For this review, take the finished solid that the model builds, in its own axes (mm). Face numbers are marked on the shaded views. A direction names the side the tool comes from. Round coordinates to 2 decimals unless told otherwise and drop trailing zeros. Order: outer loops, then holes, each group sorted by start corner. A loop starts at its lowest first (then second) coordinate and runs counter-clockwise, first axis right, second up. Notation, with made-up numbers: (14.5, 26.5) - (72.5, 26.5) arc R33 ccw to (72.5, 64.5) - close; hole circle Ø1 at (-26.75, 63). An arc over 180 degrees is marked (long way). One line per item, written item: value.
Autodesk Inventor part; units mm, degrees
ref_plane "YZ Plane" through (0, 0, 0) normal (1, 0, 0) x (0, 1, 0)
ref_plane "XZ Plane" through (0, 0, 0) normal (0, 1, 0) x (-1, 0, 0)
ref_plane "XY Plane" through (0, 0, 0) normal (0, 0, 1) x (1, 0, 0)
sketch "Sketch1" plane through (0, 0, 0) normal (0, 1, 0) x (-1, 0, 0)
  circle A0 centre (0, 0) radius 61.087
  circle A1 centre (0, 0) radius 88.9
  dimension "d0" = 122.174
  dimension "d1" = 177.8
extrude "Extrusion1" add sketch "Sketch1" along normal blind 5.08
sketch "Sketch2" plane through (0, 5.08, 0) normal (0, 1, 0) x (1, 0, 0)
  circle A0 centre (0, 0) radius 61.087
  circle A1 centre (0, 0) radius 66.167
  dimension "d4" = 132.334
  dimension "d5" = 122.174
extrude "Extrusion2" add sketch "Sketch2" along normal blind 38.354
sketch "Sketch3" plane through (0, 5.08, 0) normal (0, 1, 0) x (1, 0, 0)
  circle A0 centre (0, 0) radius 66.167
  circle A1 centre (0, 0) radius 88.9
  line L0 (66.167, 0) -> (88.9, 0) construction
  line L1 (66.167, 0) -> (77.5335, 0)
  circle A2 centre (77.5335, 0) radius 3.175
  point P0 (80.7085, 0)
  dimension "d10" = 6.35
  dimension "d8" = 22.733
  dimension "d9" = 11.3665
  dimension "d11" = 8.1915
hole "Hole1" at (77.5335, 5.08, 0) direction (0, -1, 0) diameter 6.35 end through all
pattern_circular "Circular Pattern1" count 6 over 360 about axis through (0, -10, 0) along (0, 1, 0) of "Hole1"
sketch "Sketch4" plane through (0, 5.08, 0) normal (0, 1, 0) x (1, 0, 0)
  circle A0 centre (0, 0) radius 66.167
  line L0 (43.7225, 49.663) -> (63.9658, 61.7381)
  circle A1 centre (0, 0) radius 88.9
  line L1 (64.5029, 14.7462) -> (84.7557, 26.827)
  arc A2 (64.5029, 14.7462) -> (41.6667, 51.4) centre (0, 0) ccw
  arc A3 (81.2449, 36.0899) -> (63.9658, 61.7381) centre (0, 0) ccw
  circle A4 centre (77.5335, 0) radius 3.175
  circle A5 centre (38.7668, 67.146) radius 3.175
extrude "Extrusion3" add sketch "Sketch4" along normal blind 38.354 contours A0 L0 A1 L1 picked at (52.8659, 51.2219)
sketch "Sketch5" plane through (72.0744, 43.434, -52.0431) normal (0.8107358, 0, -0.5854122) x (0, 1, 0)
  circle A0 centre (-18.8086, 0) radius 3.175
  point P0 (-43.434, 0)
  dimension "d24" = 6.35
properties part number "flangev3"
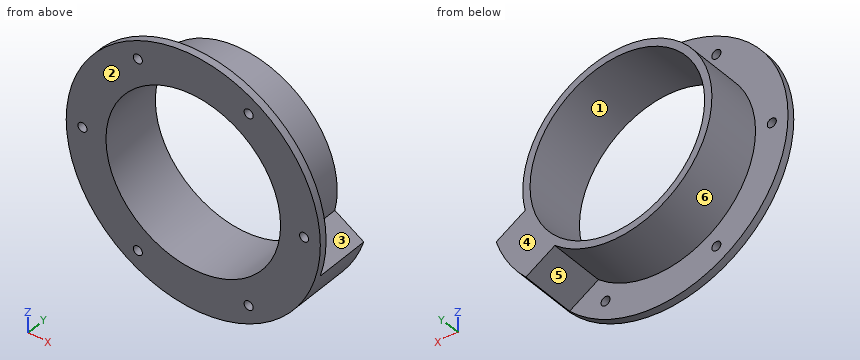
Item 1: Take a section at C-C (y = 24). Write out the cut boundary in (x, z).
Returned:
outline: (43.72, -49.66) - (63.97, -61.74) arc R88.9 ccw to (84.76, -26.83) - (64.5, -14.75) arc R66.17 ccw (long way) to start; hole circle Ø122.17 at (0, 0)
Item 2: The part is to be moulded in two halves that separate along X. For the marked faces 1, 2 and 3, say which applies: +X half, -X half, draft (parallel to the pull), parting line (faces both ways), or undercut.
Returned:
face 1: undercut
face 2: draft
face 3: +X half
Item 3: Wall thickness on line 1 (X direction, y = 3.5, z = 0); line 2 (X direction, y = 27.5, z = -54.5); line 3 (Z direction, x = 0, y = 33.5): over which ranges is each line inside the solid? List them lowest first.
Returned:
line 1: -88.9 to -80.71, -74.36 to -61.09, 61.09 to 74.36, 80.71 to 88.9
line 2: -37.52 to -27.59, 27.59 to 37.52, 51.83 to 70.24
line 3: -66.17 to -61.09, 61.09 to 66.17
Item 4: Machinability: for the marked faces 4, 5 and 6, which of the approach directions +Z, -Z, +X, -X, +Y, -Y give a long, thin tool a straight path to every point of the face, cutting with its end or side? Answer none if there is none.
Returned:
face 4: +Z, -Z, +X, -X, +Y
face 5: -Z, +Y
face 6: +Y
Item 5: Take a section at A-A (z = -56). Write out the cut boundary in (x, y), plus the area to 3 significant figures.
Returned:
outline: (-69.04, 0) - (-24.41, 0) - (-24.41, 43.43) - (-35.24, 43.43) - (-35.24, 5.08) - (-69.04, 5.08) - close; (24.41, 0) - (69.04, 0) - (69.04, 43.43) - (54.35, 43.43) - (54.35, 5.08) - (35.24, 5.08) - (35.24, 43.43) - (24.41, 43.43) - close
area: 1,850 mm^2
Item 6: For P1, Ø5.5, axis at x = -77.53, z = 0, coming from the +Y side; P2, Ø4, axis at y = 35, z = -26, coming from the +X side; P3, Ø4, axis at y = 21.5, z = -51, coming from the +X side; P4, Ø5, axis at x = 50, z = -67.5, coming from the +Y side, all flat-tipped, find the tip position at first contact; note any pin that passes through.
Returned:
P1: through
P2: x = 84.76
P3: x = 74.18
P4: y = 5.08
